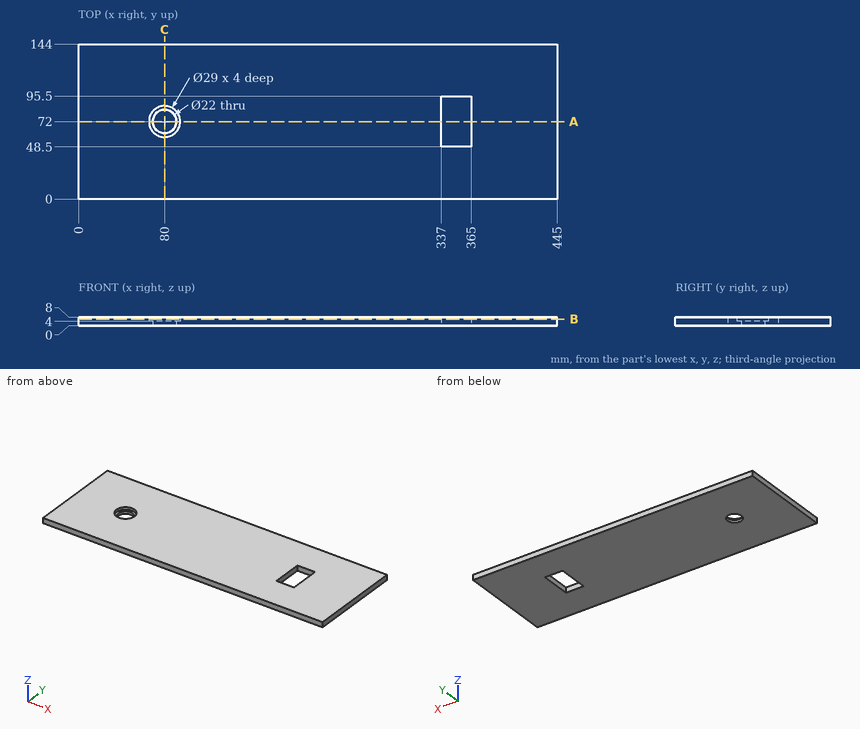
Input: dimensioned drawing with shaded views. Units: mm. Origin: part minimum x, y, z. Give positions to 0.01 mm unless a question says otherwise; leave off trailing zeros. Loops run counter-clockwise (first coordinate to the right, second up) from the corner with the lowest first, then second, coordinate; pieces in that order, holes last. Notation, with made-up numbers: (73, -28) -> (112, -28) arc R25 cw to (112, -12) -> close; hole circle Ø7 at (31.5, 65.5). An arc over 180 degrees is marked (long way). Use a Markdown table: item, result. Add a question column.
1) First-contact query: pin 1 (4 mm diameter, centred on y = 120.5, z = 3.5, fed in from -X). Flat tip, straight axial feed; report the tip coordinate or a pass-through.
2) Line query: line 1 along X through (y, z) = (71, 0.5); line 2 along Y through (x, z) = (80, 6.35); line 3 along Y through (x, z) = (80, 1.5). Output: solid intervals per line, ascending. Write a range as [from, to].
3) Section query B-B, the plane z = 6. Return the cut outline in (x, y).
4) Section query A-A, the plane y = 72. Return the cut outline in (x, z).
5) Section query C-C, the plane x = 80. Return the cut outline in (y, z), then the cut area to 3 significant figures.
Numbers:
| question | item | result |
|---|---|---|
| 1 | pin 1 | stops at x = 0 |
| 2 | line 1 | x = [0, 69.05], [90.95, 337], [365, 445] |
| 2 | line 2 | y = [0, 57.5], [86.5, 144] |
| 2 | line 3 | y = [0, 61], [83, 144] |
| 3 | outline | (0, 0) -> (445, 0) -> (445, 144) -> (0, 144) -> close; hole circle Ø29 at (80, 72); hole (337, 48.5) -> (365, 48.5) -> (365, 95.5) -> (337, 95.5) -> close |
| 4 | outline | (0, 0) -> (69, 0) -> (69, 4) -> (65.5, 4) -> (65.5, 8) -> (0, 8) -> close; (91, 0) -> (337, 0) -> (337, 8) -> (94.5, 8) -> (94.5, 4) -> (91, 4) -> close; (365, 0) -> (445, 0) -> (445, 8) -> (365, 8) -> close |
| 5 | outline | (0, 0) -> (61, 0) -> (61, 4) -> (57.5, 4) -> (57.5, 8) -> (0, 8) -> close; (83, 0) -> (144, 0) -> (144, 8) -> (86.5, 8) -> (86.5, 4) -> (83, 4) -> close |
| 5 | area | 948 mm2 |
